Check sheet for the modelled part. Datum: model origin and axes. Units: mm. Face numbers are marked on the shaded views. Round coordinates to 2 decimals unless told otherwise and drop trailing zeros. Order: outer loops, then holes, each group sorted by start corner. A loop starts at its lowest first (then second) coordinate and runs counter-clockwise, first axis right, second up. Notation, with made-up numbers: (81.5, -20.75) -> (118.5, -20.75) arc R11 cw to (118.5, -16.75) -> close; hole circle Ø7 at (18, 5.5). An arc over 180 degrees is marked (long way). Answer in a Markdown table with one row per item. Add a question column.
1. Sectioned sample at D-D, the plane y = 18. Record the boundary of the cut face in (x, z), then the cut area to 3 significant figures.
2. Material ranges on L1, parallel to Y at x = -15.5, z = 9.75; L2, parallel to Y at x = 13.5, z = 5.5; L3, parallel to X at y = -9, z = 5.5, recorded low to high. Write a range as from..to.
3. Sectioned sample at B-B, the plane x = -25.5. Record the boundary of the cut face in (y, z).
4. Draft check along Y on the marked faces 1, 2 and 3. Enter one of: +Y half, -Y half, draft (parallel to the pull), parting line (faces both ways), or undercut.
5. Sectioned sample at A-A, the plane y = 0. Record the boundary of the cut face in (x, z), then the cut area to 3 significant figures.
6. Depth check by flat-ended pin: P1, Ø1, axis at x = -38.5, z = 5.5, coming from the -Y side. Enter the tip coordinate at first touch or a pass-through.
7. Sectioned sample at C-C, the plane x = 7. Record the boundary of the cut face in (y, z).
```python
from build123d import *

# Parameters (mm, degrees)
SCHIZZO2_R                                       = 60
SCHIZZO2_R_2                                     = 48
ESTRUSIONE_ESTRUSIONE1_DEPTH                     = 10
FORO_SVASATO_PER_VITE_M4_1_D                     = 4.3
FORO_SVASATO_PER_VITE_M4_1_DEPTH                 = 28.902765847
FORO_SVASATO_PER_VITE_M4_1_CSINK_D               = 9.4
FORO_SVASATO_PER_VITE_M4_1_CSINK_ANGLE           = 90
FORO_SVASATO_PER_VITE_M4_1_ON_FACE_2_D           = 4.3
FORO_SVASATO_PER_VITE_M4_1_ON_FACE_2_DEPTH       = 28.902765847
FORO_SVASATO_PER_VITE_M4_1_ON_FACE_2_CSINK_D     = 9.4
FORO_SVASATO_PER_VITE_M4_1_ON_FACE_2_CSINK_ANGLE = 90


with BuildPart() as part:
    # Schizzo2 → Estrusione-Estrusione1 (new body)
    with BuildSketch(Plane.XY):
        Circle(SCHIZZO2_R)
        Circle(SCHIZZO2_R_2, mode=Mode.SUBTRACT)
        with BuildLine():
            ThreePointArc((-54.333327729, 14.558571287), (-56.25, 0), (-54.333327729, -14.558571287))
            ThreePointArc((-54.333327729, -14.558571287), (-51.577651768, -16.149561545), (-49.98666151, -13.393885584))
            ThreePointArc((-49.98666151, -13.393885584), (-51.75, 0), (-49.98666151, 13.393885584))
            ThreePointArc((-49.98666151, 13.393885584), (-51.577651768, 16.149561545), (-54.333327729, 14.558571287))
        make_face(mode=Mode.SUBTRACT)
        with BuildLine():
            ThreePointArc((-13.393885584, -49.98666151), (-16.149561545, -51.577651768), (-14.558571287, -54.333327729))
            ThreePointArc((-14.558571287, -54.333327729), (0, -56.25), (14.558571287, -54.333327729))
            ThreePointArc((14.558571287, -54.333327729), (16.149561545, -51.577651768), (13.393885584, -49.98666151))
            ThreePointArc((13.393885584, -49.98666151), (0, -51.75), (-13.393885584, -49.98666151))
        make_face(mode=Mode.SUBTRACT)
        with BuildLine():
            ThreePointArc((13.393885584, 49.98666151), (16.149561545, 51.577651768), (14.558571287, 54.333327729))
            ThreePointArc((14.558571287, 54.333327729), (0, 56.25), (-14.558571287, 54.333327729))
            ThreePointArc((-14.558571287, 54.333327729), (-16.149561545, 51.577651768), (-13.393885584, 49.98666151))
            ThreePointArc((-13.393885584, 49.98666151), (0, 51.75), (13.393885584, 49.98666151))
        make_face(mode=Mode.SUBTRACT)
        with BuildLine():
            ThreePointArc((54.333327729, 14.558571287), (51.577651768, 16.149561545), (49.98666151, 13.393885584))
            ThreePointArc((49.98666151, 13.393885584), (51.75, 0), (49.98666151, -13.393885584))
            ThreePointArc((49.98666151, -13.393885584), (51.577651768, -16.149561545), (54.333327729, -14.558571287))
            ThreePointArc((54.333327729, -14.558571287), (56.25, 0), (54.333327729, 14.558571287))
        make_face(mode=Mode.SUBTRACT)
    extrude(amount=ESTRUSIONE_ESTRUSIONE1_DEPTH)

    # Foro svasato per Vite M4-1
    with Locations(Plane(origin=(-16.41696688, -45.105245798, 5), x_dir=(0.939692620786, -0.342020143326, 0), z_dir=(0.342020143326, 0.939692620786, 0))):
        with Locations((0, 0)):
            CounterSinkHole(FORO_SVASATO_PER_VITE_M4_1_D / 2, FORO_SVASATO_PER_VITE_M4_1_CSINK_D / 2, depth=FORO_SVASATO_PER_VITE_M4_1_DEPTH, counter_sink_angle=FORO_SVASATO_PER_VITE_M4_1_CSINK_ANGLE)

    # Foro svasato per Vite M4-1 on face 2
    with Locations(Plane(origin=(16.41696688, -45.105245798, 5), x_dir=(0.939692711209, 0.342019894889, 0), z_dir=(-0.342019894889, 0.939692711209, 0))):
        with Locations((0, 0)):
            CounterSinkHole(FORO_SVASATO_PER_VITE_M4_1_ON_FACE_2_D / 2, FORO_SVASATO_PER_VITE_M4_1_ON_FACE_2_CSINK_D / 2, depth=FORO_SVASATO_PER_VITE_M4_1_ON_FACE_2_DEPTH, counter_sink_angle=FORO_SVASATO_PER_VITE_M4_1_ON_FACE_2_CSINK_ANGLE)


solid = part.part
```
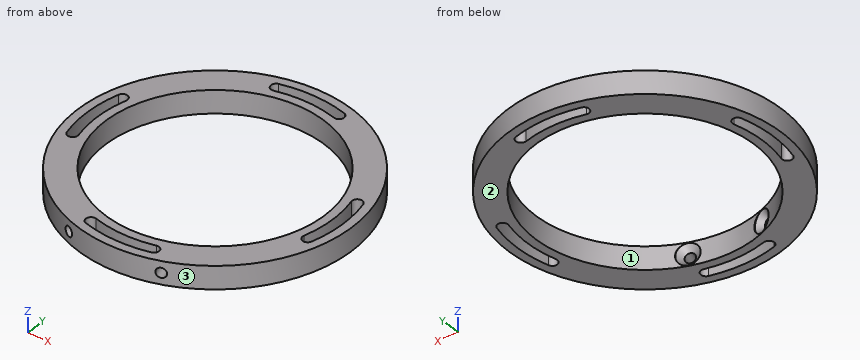
Answer key:
| question | item | result |
|---|---|---|
| 1 | outline | (-57.24, 0) -> (-44.5, 0) -> (-44.5, 10) -> (-57.24, 10) -> close; (44.5, 0) -> (57.24, 0) -> (57.24, 10) -> (44.5, 10) -> close |
| 1 | area | 255 mm² |
| 2 | L1 | y = -57.96..-53.82, -50.5..-45.43, 45.43..50.5, 53.82..57.96 |
| 2 | L2 | y = -58.46..-54.61, -49.96..-47.38, 46.06..49.96, 54.61..58.46 |
| 2 | L3 | x = -59.32..-55.53, -50.96..-47.15, 47.15..50.96, 55.53..59.32 |
| 3 | outline | (-54.31, 0) -> (-40.67, 0) -> (-40.67, 10) -> (-54.31, 10) -> close; (40.67, 0) -> (54.31, 0) -> (54.31, 10) -> (40.67, 10) -> close |
| 4 | face 1 | undercut |
| 4 | face 2 | draft |
| 4 | face 3 | parting line |
| 5 | outline | (-60, 0) -> (-56.25, 0) -> (-56.25, 10) -> (-60, 10) -> close; (-51.75, 0) -> (-48, 0) -> (-48, 10) -> (-51.75, 10) -> close; (48, 0) -> (51.75, 0) -> (51.75, 10) -> (48, 10) -> close; (56.25, 0) -> (60, 0) -> (60, 10) -> (56.25, 10) -> close |
| 5 | area | 150 mm² |
| 6 | P1 | stops at y = -46.43 |
| 7 | outline | (-59.59, 0) -> (-55.81, 0) -> (-55.81, 10) -> (-59.59, 10) -> close; (-51.27, 0) -> (-47.49, 0) -> (-47.49, 10) -> (-51.27, 10) -> close; (47.49, 0) -> (51.27, 0) -> (51.27, 10) -> (47.49, 10) -> close; (55.81, 0) -> (59.59, 0) -> (59.59, 10) -> (55.81, 10) -> close |
